from build123d import *

# Parameters (mm, degrees)
BOSS_EXTRU_2_DEPTH      = 2
CHANFREIN2_SIZE         = 2
ESQUISSE6_W             = 2.5
ESQUISSE6_H             = 7.4
BOSS_EXTRU_5_DEPTH      = 3
ENL_V_MAT_EXTRU_5_DEPTH = 1.4
ENL_V_START             = -1.4
ENL_V_MAT_EXTRU_6_DEPTH = 1.4


with BuildPart() as part:
    # Esquisse1 → Boss.-Extru.2 (new body)
    with BuildSketch(Plane(origin=(0, 0, 0), x_dir=(1, 0, 0), z_dir=(0, 1, 0))):
        Polygon((0, 12.2), (0, 0), (120, 0), (120, 12.2), (65, 12.2), (65, 9.2), (55, 9.2), (55, 12.2), align=None)
    extrude(amount=BOSS_EXTRU_2_DEPTH)

    # Chanfrein2
    chanfrein2_edges = [part.edges().sort_by_distance(p)[0] for p in [
        (92.5, 0, -12.2),
        (27.5, 0, -12.2),
        (60, 0, -9.2),
        (60, 0, 0),
    ]]
    chamfer(chanfrein2_edges, length=CHANFREIN2_SIZE - 0.0001)  # a hair under: the kernel refuses the full size

    # Esquisse6 → Boss.-Extru.5 (add)
    with BuildSketch(Plane.XZ):
        with Locations((1.25, -6.1)):
            Rectangle(ESQUISSE6_W, ESQUISSE6_H)
        with Locations((118.75, -6.1)):
            Rectangle(ESQUISSE6_W, ESQUISSE6_H)
    extrude(amount=BOSS_EXTRU_5_DEPTH)

    # Esquisse9 → Enlèv. mat.-Extru.5 (cut)
    with BuildSketch(Plane.ZY):
        with BuildLine():
            ThreePointArc((-4.2, -0.5), (-4.235817666, -0.132815816), (-4.341920237, 0.220524493))
            Line((-4.341920237, 0.220524493), (-7.858079763, -1.220524493))
            ThreePointArc((-7.858079763, -1.220524493), (-5.732815816, -2.364182334), (-4.2, -0.5))
        make_face()
        with BuildLine():
            Line((-7.858079763, -1.220524493), (-4.341920237, 0.220524493))
            ThreePointArc((-4.341920237, 0.220524493), (-6.820524493, 1.258079763), (-7.858079763, -1.220524493))
        make_face()
    extrude(amount=-ENL_V_MAT_EXTRU_5_DEPTH, mode=Mode.SUBTRACT)

    # Esquisse10 → Enlèv. mat.-Extru.6 (cut)
    with BuildSketch(Plane(origin=(120, 0, 0), x_dir=(0, 0, -1), z_dir=(1, 0, 0)).offset(ENL_V_START)):
        with BuildLine():
            ThreePointArc((8, -0.5), (7.964182334, -0.132815816), (7.858079763, 0.220524493))
            Line((7.858079763, 0.220524493), (4.341920237, -1.220524493))
            ThreePointArc((4.341920237, -1.220524493), (6.467184184, -2.364182334), (8, -0.5))
        make_face()
        with BuildLine():
            Line((4.341920237, -1.220524493), (7.858079763, 0.220524493))
            ThreePointArc((7.858079763, 0.220524493), (5.379475507, 1.258079763), (4.341920237, -1.220524493))
        make_face()
    extrude(amount=ENL_V_MAT_EXTRU_6_DEPTH, mode=Mode.SUBTRACT)


solid = part.part
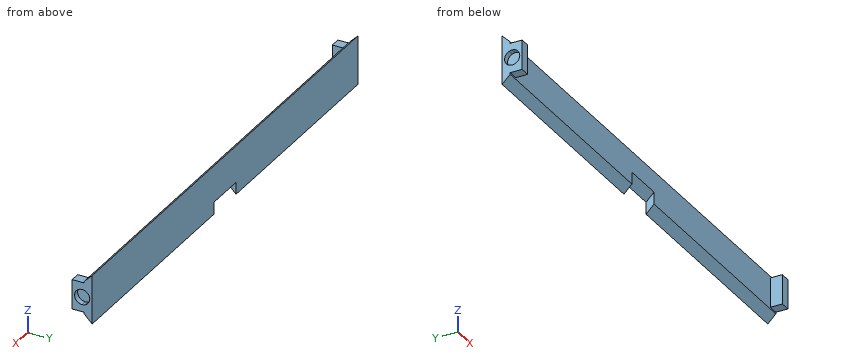
For this review, take the finished solid that the model builds, in its own axes (mm). Give positions to 0.01 mm unless a question says otherwise; leave off trailing zeros. Order: outer loops, then holes, each group sorted by start corner. A loop starts at its lowest first (then second) coordinate and runs counter-clockwise, first axis right, second up. Notation, with made-up numbers: M -32.75,-37.5 L 16.25,-37.5 A26 ccw 16.25,-9.5 Z; hole C 13,-32.75 d8. An arc over 180 degrees is marked long. Answer in a Markdown table with one row per item. Add a question column.
(1) Consider section A-A on z = -6.1. State the section outline as (x, y) points.
(2) Wall thickness on probe 1 along X at (y, z) = (-1.45, -8.5); probe 2 along X at (y, z) = (-1.05, -5.75); probe 3 along Y at (x, z) = (43, -4.25): over which ranges is each line inside the solid? List them lowest first. Write a range as [from, to].
(3) For pin 1 (2 mm diameter, centred on x = 1, y = -2, fed in from -Z); pin 2 (1 mm diameter, centred on x = 90.5, y = -1.5, fed in from -Z); pin 3 (1 mm diameter, centred on x = 49.5, z = -3, fed in from -Y); pin 4 (2 mm diameter, centred on x = 119, y = -2, fed in from +Z), all flat-tipped, find the tip position at first contact; note any pin that passes through.
Evaluation:
| question | item | result |
|---|---|---|
| 1 | outline | M 0,-3 L 2.5,-3 L 2.5,0 L 117.5,0 L 117.5,-3 L 120,-3 L 120,-2.4 L 118.6,-2.4 L 118.6,1.4 L 120,1.4 L 120,2 L 0,2 L 0,1.4 L 1.4,1.4 L 1.4,-2.4 L 0,-2.4 Z |
| 2 | probe 1 | x = [0, 2.5], [117.5, 120] |
| 2 | probe 2 | x = [1.4, 2.5], [117.5, 118.6] |
| 2 | probe 3 | y = [0, 2] |
| 3 | pin 1 | stops at z = -9.8 |
| 3 | pin 2 | passes through |
| 3 | pin 3 | stops at y = 0 |
| 3 | pin 4 | stops at z = -2.4 |
